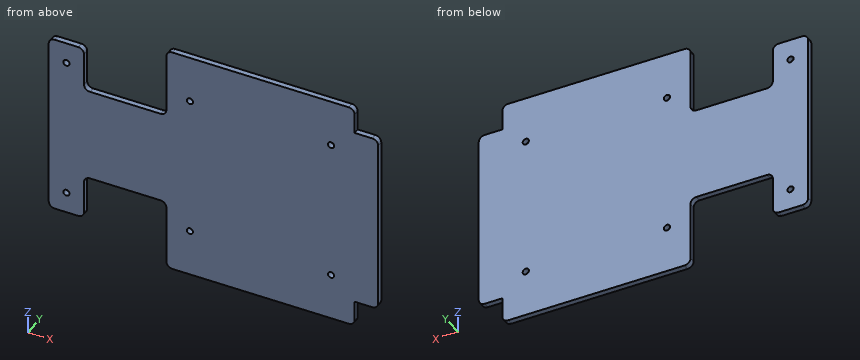
```python
from build123d import *

# Parameters (mm, degrees)
BOSS_EXTRUDE1_DEPTH = 6.35
SKETCH2_R           = 3.3655
CUT_EXTRUDE1_DEPTH  = 262.586090036


with BuildPart() as part:
    # Sketch1 → Boss-Extrude1 (new body)
    with BuildSketch(Plane(origin=(0, 0, 0), x_dir=(1, 0, 0), z_dir=(0, 1, 0))):
        with BuildLine():
            Line((-222.25, 99.06), (-196.85, 99.06))
            ThreePointArc((-196.85, 99.06), (-192.359871939, 97.200128061), (-190.5, 92.71))
            Line((-190.5, 92.71), (-190.5, 57.15))
            ThreePointArc((-190.5, 57.15), (-188.640128061, 52.659871939), (-184.15, 50.8))
            Line((-184.15, 50.8), (-107.95, 50.8))
            ThreePointArc((-107.95, 50.8), (-103.459871939, 52.659871939), (-101.6, 57.15))
            Line((-101.6, 57.15), (-101.6, 120.65))
            ThreePointArc((-101.6, 120.65), (-99.740128061, 125.140128061), (-95.25, 127))
            Line((-95.25, 127), (95.25, 127))
            ThreePointArc((95.25, 127), (99.740128061, 125.140128061), (101.6, 120.65))
            Line((101.6, 120.65), (101.6, 99.06))
            Line((101.6, 99.06), (120.65, 99.06))
            ThreePointArc((120.65, 99.06), (125.14012806, 97.200128061), (127, 92.71))
            Line((127, 92.71), (127, -92.71))
            ThreePointArc((127, -92.71), (125.14012806, -97.200128061), (120.65, -99.06))
            Line((120.65, -99.06), (101.6, -99.06))
            Line((101.6, -99.06), (101.6, -120.65))
            ThreePointArc((101.6, -120.65), (99.740128061, -125.140128061), (95.25, -127))
            Line((95.25, -127), (-95.25, -127))
            ThreePointArc((-95.25, -127), (-99.740128061, -125.140128061), (-101.6, -120.65))
            Line((-101.6, -120.65), (-101.6, -57.15))
            ThreePointArc((-101.6, -57.15), (-103.459871939, -52.659871939), (-107.95, -50.8))
            Line((-107.95, -50.8), (-184.15, -50.8))
            ThreePointArc((-184.15, -50.8), (-188.640128061, -52.659871939), (-190.5, -57.15))
            Line((-190.5, -57.15), (-190.5, -92.71))
            ThreePointArc((-190.5, -92.71), (-192.359871939, -97.200128061), (-196.85, -99.06))
            Line((-196.85, -99.06), (-222.25, -99.06))
            ThreePointArc((-222.25, -99.06), (-226.740128061, -97.200128061), (-228.6, -92.71))
            Line((-228.6, -92.71), (-228.6, 92.71))
            ThreePointArc((-228.6, 92.71), (-226.740128061, 97.200128061), (-222.25, 99.06))
        make_face()
    extrude(amount=BOSS_EXTRUDE1_DEPTH)

    # Sketch2 → Cut-Extrude1 (cut, through all)
    with BuildSketch(Plane(origin=(0, 6.35, 0), x_dir=(1, 0, 0), z_dir=(0, 1, 0))):
        with Locations(Location((-76.2, 76.2, 0), (0, 0, 270))):
            Circle(SKETCH2_R)
        with Locations(Location((76.2, 76.2, 0), (0, 0, 270))):
            Circle(SKETCH2_R)
        with Locations(Location((-76.2, -76.2, 0), (0, 0, 270))):
            Circle(SKETCH2_R)
        with Locations(Location((76.2, -76.2, 0), (0, 0, 270))):
            Circle(SKETCH2_R)
        with Locations(Location((-209.55, 76.2, 0), (0, 0, 270))):
            Circle(SKETCH2_R)
        with Locations(Location((-209.55, -76.2, 0), (0, 0, 270))):
            Circle(SKETCH2_R)
    extrude(amount=-CUT_EXTRUDE1_DEPTH, mode=Mode.SUBTRACT)


solid = part.part
```
Source: CAD feature listing. Evaluate the final solid. Frame: model axes, mm. Coordinates: 2 decimals unless noted, no trailing zeros. Loops run counter-clockwise (first coordinate to the right, second up) from the corner with the lowest first, then second, coordinate; pieces in that order, holes last. Notation, with made-up numbers: M 48.25,3 L 74.25,3 A20 cw 74.25,16 Z; hole C -0.5,10.5 d11. An arc over 180 degrees is marked long. Put each result on its own line as item: value. Start each with the question number.
1) Cut plane A-A on z = -64.5. Return the cut outline in (x, y).
2) Cut plane B-B on x = -178. Return the cut outline in (y, z), then the cut area to 3 significant figures.
3) Ray query, L1, parallel to Z at x = -209.55, y = 5.25; L2, parallel to X at y = 2, z = -76.2; L3, parallel to X at y = 3.25, z = -99.5. Return the intervals inside material, ascending. Write a range as from..to.
4) Cut plane C-C on z = -109. Return the cut outline in (x, y).
5) Contact query for flat-ended pins moving along their axis: pin 1 Ø2 at (x, y) = (-123, 1) entering from +Z; pin 2 Ø6 at (x, z) = (-76.2, 76.2) entering from +Y; pin 3 Ø3 at (x, y) = (-205.5, 2) entering from -Z; pin 4 Ø3 at (y, z) = (2.5, -114) entering from +X. Output: stop coordinate, or through.
The answers:
1. outline: M -228.6,0 L -190.5,0 L -190.5,6.35 L -228.6,6.35 Z; M -101.6,0 L 127,0 L 127,6.35 L -101.6,6.35 Z
2. outline: M 0,-50.8 L 6.35,-50.8 L 6.35,50.8 L 0,50.8 Z
2. area: 645 mm²
3. L1: z = -99.06..-79.57, -72.83..72.83, 79.57..99.06
3. L2: x = -228.6..-212.92, -206.18..-190.5, -101.6..-79.57, -72.83..72.83, 79.57..127
3. L3: x = -101.6..101.6
4. outline: M -101.6,0 L 101.6,0 L 101.6,6.35 L -101.6,6.35 Z
5. pin 1: stops at z = 50.8
5. pin 2: passes through
5. pin 3: stops at z = -99.06
5. pin 4: stops at x = 101.6
